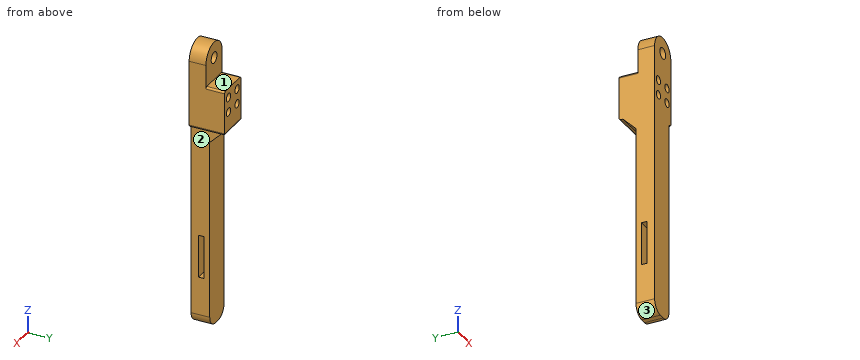
from build123d import *

# Parameters (mm, degrees)
CYLINDER029_R          = 2.2
CYLINDER029_DEPTH      = 26
CYLINDER029_ROLL_ANGLE = -90
ARRAY001_X_COUNT       = 2
ARRAY001_X_PITCH       = 8
ARRAY001_Z_COUNT       = 2
ARRAY001_Z_PITCH       = 9
BOX015_W               = 23
BOX015_H               = 3
BOX015_DEPTH           = 20
BOX011_W               = 130
BOX011_H               = 10
BOX011_DEPTH           = 15
SKETCH003_R            = 3
PAD003_DEPTH           = 9
FILLET003_R            = 1
BOX013_W               = 24
BOX013_H               = 10
BOX013_DEPTH           = 17
FILLET_R               = 1
CHAMFER_SIZE           = 7
FILLET004_R            = 6
FILLET004_PITCH_ANGLE  = 90


with BuildPart() as obj1:
    # Cylinder029 → Cylinder029 (new body)
    with BuildSketch(Plane.XY):
        Circle(CYLINDER029_R)
    extrude(amount=CYLINDER029_DEPTH)


with BuildPart() as obj1_1:
    # Cylinder029 roll: moved
    add(obj1.part.rotate(Axis((0, 0, 0), (1, 0, 0)), CYLINDER029_ROLL_ANGLE))


with BuildPart() as obj1_2:
    # Cylinder029 placement: moved
    add(obj1_1.part.moved(Location((202, 0, 4))))

    # Array001 X: obj1_2


with BuildPart() as obj1_3:
    add(obj1_2.part)
    with Locations(*[(i * ARRAY001_X_PITCH, 0, 0) for i in range(1, ARRAY001_X_COUNT)]):
        add(obj1_2.part)

    # Array001 Z: obj1_2


with BuildPart() as obj1_4:
    add(obj1_3.part)
    with Locations(*[(0, 0, i * ARRAY001_Z_PITCH) for i in range(1, ARRAY001_Z_COUNT)]):
        add(obj1_3.part)


with BuildPart() as obj2:
    # Box015 → Box015 (new body)
    with BuildSketch(Plane(origin=(280.5, 5, 0), x_dir=(1, 0, 0), z_dir=(0, 0, 1))):
        with Locations((11.5, 1.5)):
            Rectangle(BOX015_W, BOX015_H)
    extrude(amount=BOX015_DEPTH)


with BuildPart() as base_tibia:
    # Box011 → Box011 (new body)
    with BuildSketch(Plane(origin=(200, 1.5, 0), x_dir=(1, 0, 0), z_dir=(0, 0, 1))):
        with Locations((65, 5)):
            Rectangle(BOX011_W, BOX011_H)
    extrude(amount=BOX011_DEPTH)


with BuildPart() as obj3:
    # Sketch003 → Pad003 (new body)
    with BuildSketch(Plane(origin=(221, 10.5, 0), x_dir=(1, 0, 0), z_dir=(0, -1, 0))):
        with BuildLine():
            Line((0, 17), (-36, 17))
            ThreePointArc((-36, 17), (-44.500015, 8.5), (-36, 0))
            Line((-36, 0), (0, 0))
            Line((0, 0), (0, 17))
        make_face()
        with Locations((-36.000015, 8.5)):
            Circle(SKETCH003_R, mode=Mode.SUBTRACT)
    extrude(amount=PAD003_DEPTH)

    # Fillet003
    fillet003_edges = [obj3.edges().sort_by_distance(p)[0] for p in [
        (221, 6, 17),
        (221, 6, 0),
    ]]
    fillet(fillet003_edges, radius=FILLET003_R)

    # Fusion008: union Base_tibia
    add(base_tibia.part)


with BuildPart() as obj3_1:
    # Fusion008 placement: moved
    add(obj3.part.moved(Location((0, -0.5, 0))))

    # Cut010: cut obj2
    add(obj2.part, mode=Mode.SUBTRACT)


with BuildPart() as obj4:
    # Box013 → Box013 (new body)
    with BuildSketch(Plane(origin=(197, 10, 0), x_dir=(1, 0, 0), z_dir=(0, 0, 1))):
        with Locations((12, 5)):
            Rectangle(BOX013_W, BOX013_H)
    extrude(amount=BOX013_DEPTH)

    # Fillet
    fillet_edges = [obj4.edges().sort_by_distance(p)[0] for p in [
        (197, 15, 17),
        (197, 15, 0),
        (221, 15, 17),
        (221, 20, 8.5),
    ]]
    fillet(fillet_edges, radius=FILLET_R)

    # Fusion009003008: union obj3
    add(obj3_1.part)

    # Chamfer
    chamfer_edges = [obj4.edges().sort_by_distance(p)[0] for p in [
        (221, 11, 7.5),
    ]]
    chamfer(chamfer_edges, length=CHAMFER_SIZE)

    # Cut011: cut obj1
    add(obj1_4.part, mode=Mode.SUBTRACT)

    # Fillet004
    fillet004_edges = [obj4.edges().sort_by_distance(p)[0] for p in [
        (330, 6, 0),
        (330, 6, 15),
    ]]
    fillet(fillet004_edges, radius=FILLET004_R)


with BuildPart() as obj4_1:
    # Fillet004 pitch: moved
    add(obj4.part.rotate(Axis((0, 0, 0), (0, 1, 0)), FILLET004_PITCH_ANGLE))


with BuildPart() as obj4_2:
    # Fillet004 placement: moved
    add(obj4_1.part.moved(Location((359, 67, 326))))


solid = obj4_2.part
Source: CAD feature listing. Evaluate the final solid. Frame: model axes, mm. Face numbers are marked on the shaded views. A direction names the side the tool comes from. Round coordinates to 2 decimals unless told otherwise and drop trailing zeros. Loops run counter-clockwise (first coordinate to the right, second up) from the corner with the lowest first, then second, coordinate; pieces in that order, holes last. Notation, with made-up numbers: (69.5, -22.75) -> (76.5, -22.75) arc R30 cw to (76.5, 3.25) -> close; hole circle Ø8 at (20, -36). An arc over 180 degrees is marked (long way). Answer as a JSON object with one key per item and string values. Group by question number.
Q1. Section query C-C (x = 363). Output: boundary loops of the cut face in (y, z).
Q2. Contact query for flat-ended pins moving along their axis: P1, Ø10, axis at x = 373.5, y = 77.5, coming from the +Z side; P2, Ø2, axis at x = 363, z = 94, coming from the +Y side; P3, Ø5, axis at y = 79, z = 67, coming from the +X side. Output: stop coordinate, or through.
Q3. Access query for the marked faces 1, 2 and 3. Directions: +Z, -Z, +X, -X, +Y, -Y. A direction counts if a zero-diameter tool reaches every point of the face in a straight line with its end or side. Return the directions, or none.
Q4. Ray query, line 1 (Y direction, x = 361, z = 34); line 2 (X direction, y = 78.5, z = 116); line 3 (Z direction, x = 372.25, y = 69). Return the intervals inside material, ascending. Write a range as from..to.
Q5. Section query B-B (z = 116). Output: boundary loops of the cut face in (x, y).
Q6. Section query D-D (z = 19). Output: boundary loops of the cut face in (x, y).
Q7. Section query A-A (y = 73.75). Output: boundary loops of the cut face in (x, z), plus the area to 3 significant figures.
Completed:
{
 "1": {"outline": "(68, -3.66) -> (78, -3.66) -> (78, 98) -> (85, 105) -> (86, 105) arc R1 ccw to (87, 106) -> (87, 113.8) -> (68, 113.8) -> close; (68, 118.2) -> (87, 118.2) -> (87, 121.8) -> (68, 121.8) -> close; (68, 126.2) -> (87, 126.2) -> (87, 129) -> (77, 129) -> (77, 148.21) -> (68, 148.21) -> close; hole (72, 22.5) -> (75, 22.5) -> (75, 45.5) -> (72, 45.5) -> close"},
 "2": {"P1": "z = 149.44", "P2": "y = 78", "P3": "x = 374"},
 "3": {"face 1": "+Z, +X, -X, +Y", "face 2": "-Z, +X, +Y, -Y", "face 3": "-Z, -X, +Y, -Y"},
 "4": {"line 1": "68..72, 75..78", "line 2": "359..360.8, 365.2..369.8, 374.2..376", "line 3": "-2.24..113.81, 118.19..121.81, 126.19..148.05"},
 "5": {"outline": "(359, 68) -> (360.8, 68) -> (360.8, 87) -> (359, 87) -> close; (365.2, 68) -> (369.8, 68) -> (369.8, 87) -> (365.2, 87) -> close; (374.2, 68) -> (376, 68) -> (376, 87) -> (374.2, 87) -> close"},
 "6": {"outline": "(359, 68) -> (374, 68) -> (374, 78) -> (359, 78) -> close"},
 "7": {"outline": "(359, 2) arc R6 ccw to (365, -4) -> (368, -4) arc R6 ccw to (374, 2) -> (374, 22.5) -> (359, 22.5) -> close; (359, 45.5) -> (374, 45.5) -> (374, 105) -> (375, 105) arc R1 ccw to (376, 106) -> (376, 141) arc R8.5 ccw to (359, 141) -> close; hole circle Ø4.4 at (363, 116); hole circle Ø4.4 at (363, 124); hole circle Ø6 at (367.5, 141); hole circle Ø4.4 at (372, 116); hole circle Ø4.4 at (372, 124)", "area": "1,910 mm²"}
}
